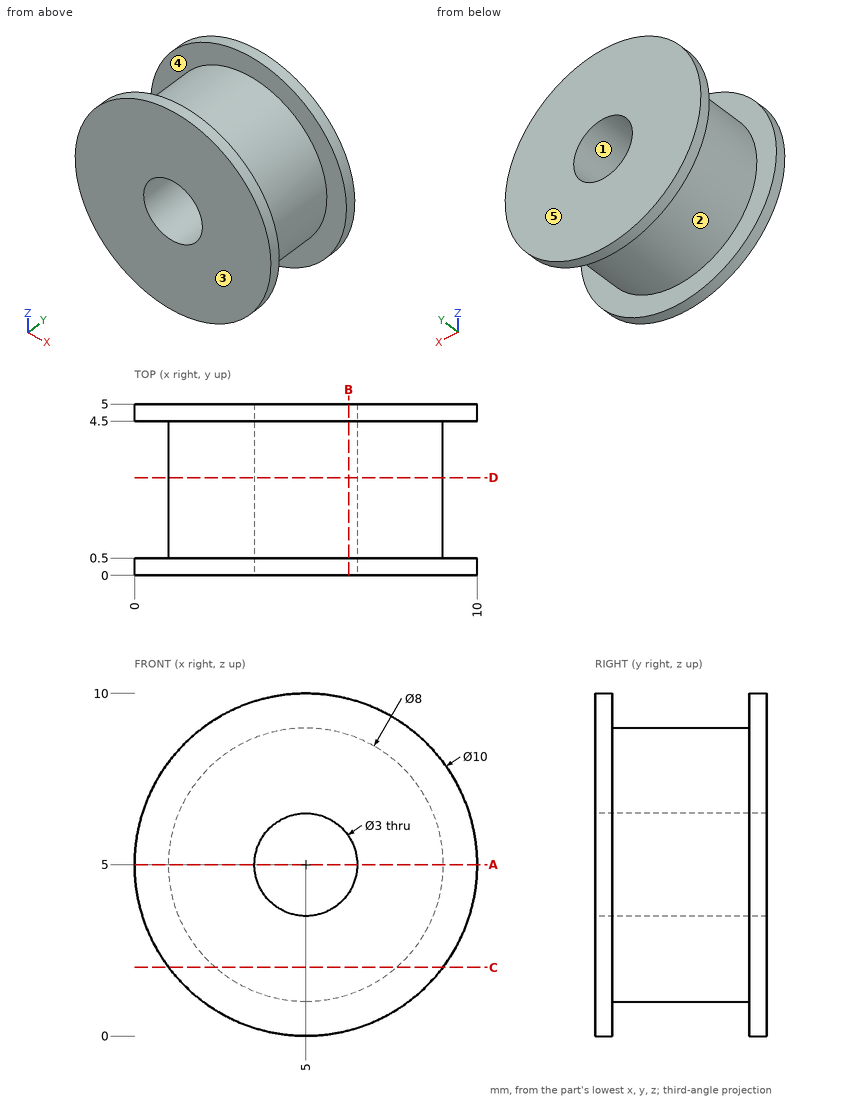
Study the drawing (mm; zero at the part's minimum x, y, z) and answer. A direction names the side the tool comes from. Coordinates: 2 decimals unless noted, no trailing zeros. Order: outer loops, then holes, each group sorted by start corner. A loop starts at its lowest first (then second) coordinate and runs counter-clockwise, first axis right, second up. Notation, with made-up numbers: M 64,63.25 L 73,63.25 A6 ccw 73,73.25 Z; hole C -22.75,-0.5 d3. An arc over 180 degrees is marked long. Answer as a JSON object with one key per item and string values. Group by question number.
1. Section A-A on z = 5 is taken. Write down the section's boundary in (x, y).
2. Section B-B on x = 6.25 is taken. Write down the section's boundary in (y, z).
3. A tool of negligible diameter and unlimited length cuts with its end or side. For the marked faces 4 and 5, from which of +Z, -Z, +X, -X, +Y, -Y can it reach the whole face along a straight path? Write none if from no direction.
4. Straight lines are drawn through the part: line 1 (Y direction, x = 4, z = 9.75); line 2 (X direction, y = 3.5, z = 5); line 3 (Z direction, x = 5.25, y = 3.05). For each, find the intervals that lie inside material, in ascending order.
5. Section C-C on z = 2 is taken. Write down the section's boundary in (x, y).
6. Section D-D on y = 2.85 is taken. Write down the section's boundary in (x, z).
7. Determine the mould class of the marked faces 1, 2 and 3 for opening direction Z: released by +Z, released by -Z, zero draft, split by the parting line, or undercut.
Values follow:
{
 "1": {"outline": "M 0,0 L 3.5,0 L 3.5,5 L 0,5 L 0,4.5 L 1,4.5 L 1,0.5 L 0,0.5 Z; M 6.5,0 L 10,0 L 10,0.5 L 9,0.5 L 9,4.5 L 10,4.5 L 10,5 L 6.5,5 Z"},
 "2": {"outline": "M 0,0.16 L 0.5,0.16 L 0.5,1.2 L 4.5,1.2 L 4.5,0.16 L 5,0.16 L 5,4.17 L 0,4.17 Z; M 0,5.83 L 5,5.83 L 5,9.84 L 4.5,9.84 L 4.5,8.8 L 0.5,8.8 L 0.5,9.84 L 0,9.84 Z"},
 "3": {"face 4": "none", "face 5": "+Z, -Z, +X, -X, +Y"},
 "4": {"line 1": "0 to 0.5, 4.5 to 5", "line 2": "1 to 3.5, 6.5 to 9", "line 3": "1.01 to 3.52, 6.48 to 8.99"},
 "5": {"outline": "M 1,0 L 9,0 L 9,0.5 L 7.65,0.5 L 7.65,4.5 L 9,4.5 L 9,5 L 1,5 L 1,4.5 L 2.35,4.5 L 2.35,0.5 L 1,0.5 Z"},
 "6": {"outline": "C 5,5 d8; hole C 5,5 d3"},
 "7": {"face 1": "undercut", "face 2": "split by the parting line", "face 3": "zero draft"}
}
